Part model, mm, in its own coordinate system. A direction names the side the tool comes from. Coordinates: 2 decimals unless noted, no trailing zeros. Order: outer loops, then holes, each group sorted by start corner. A loop starts at its lowest first (then second) coordinate and runs counter-clockwise, first axis right, second up.
```python
from build123d import *

# Parameters (mm, degrees)
BOSS_EXTRUDE1_DEPTH = 15
SHELL1_T            = -5


with BuildPart() as part:
    # Sketch1 → Boss-Extrude1 (new body)
    with BuildSketch(Plane.XY):
        with BuildLine():
            Line((-97.924180929, -245.60870674), (-107.924180929, -245.521090808))
            ThreePointArc((-107.924180929, -245.521090808), (-140.543987168, -222.66060862), (-160.924180929, -188.436332043))
            Line((-160.924180929, -188.436332043), (-160.924180929, -159.60870674))
            Line((-160.924180929, -159.60870674), (-97.924180929, -159.60870674))
            Line((-97.924180929, -159.60870674), (-97.924180929, -245.60870674))
        make_face()
    extrude(amount=BOSS_EXTRUDE1_DEPTH)

    # Shell1
    shell1_openings = [part.faces().sort_by_distance(p)[0] for p in [
        (-125.349491383, -195.90901573, 0),
    ]]
    offset(amount=SHELL1_T, openings=shell1_openings, kind=Kind.INTERSECTION)


solid = part.part
```
(1) Pull direction Y, two halves, no side cores. Call faces 1 (the face through (-140.16, -223.07, 7.4)), 2 (the face through (-102.924, -202, 5)), 3 (the face through (-130, -159.609, 7)), 4 (the face through (-155.924, -176, 5)): +Y half, -Y half, draft (parallel to the pull), parting line (faces both ways), or undercut.
(2) Drop flat-ended pins along their axis: pin 1 (8 mm diameter, centred on x = -124.5, z = 12, fed in from -Y); pin 2 (1.5 mm diameter, centred on y = -192, z = 8.5, fed in from -X); pin 3 (5 mm diameter, centred on x = -122, z = 6.5, fed in from -Y). Give the stop position or say it passes through.
(3) Tool access for faces 5 (the face through (-160.924, -174, 7)), 6 (the face through (-130, -164.609, 5)): list every direction of +Z, -Z, +X, -X, +Y, -Y with a clear straight run to the whole face (end or side of a thin tool).
(4) Slice it at C-C, the plane x = -122.5. Give the cut face in (y, z).
(5) Slice it at A-A, the plane z = 2.5. Give the cut face in (x, y).
(6) Probe line 1 (X direction, y = -170.5, z = 3.25); line 2 (Z direction, x = -139.5, y = -170); line 3 (Y direction, x = -140.5, z = 3.75). List the from-to ranges inside material, lowest first.
(7) Slice it at B-B, the plane y = -184.5. Give the cut face in (x, z).
Here are the results:
1. face 1: -Y half
1. face 2: undercut
1. face 3: +Y half
1. face 4: undercut
2. pin 1: stops at y = -239.06
2. pin 2: stops at x = -159.92
2. pin 3: stops at y = -239.66
3. face 5: +Z, -Z, -X, +Y, -Y
3. face 6: -Z
4. outline: (-237.8, 0) - (-231.78, 0) - (-231.78, 10) - (-164.61, 10) - (-164.61, 0) - (-159.61, 0) - (-159.61, 15) - (-237.8, 15) - close
5. outline: (-160.92, -188.44) arc R95 ccw to (-107.92, -245.52) - (-97.92, -245.61) - (-97.92, -159.61) - (-160.92, -159.61) - close; hole (-155.92, -187.6) arc R90 ccw to (-106.88, -240.53) - (-102.92, -240.56) - (-102.92, -164.61) - (-155.92, -164.61) - close
6. line 1: x = -160.92 to -155.92, -102.92 to -97.92
6. line 2: z = 10 to 15
6. line 3: y = -222.71 to -215.11, -164.61 to -159.61
7. outline: (-160.92, 0) - (-155.92, 0) - (-155.92, 10) - (-102.92, 10) - (-102.92, 0) - (-97.92, 0) - (-97.92, 15) - (-160.92, 15) - close
